from build123d import *

# Parameters (mm, degrees)
SKETCH3_R   = 14.887575
SKETCH3_R_2 = 10.4648
FILLET1_R   = 4.422775


with BuildPart() as part:
    # Sketch1 → Revolve1 (revolve)
    with BuildSketch(Plane.XY):
        Polygon((-26.19375, -17.859375), (-23.22195, -14.887575), (-23.22195, -10.4648), (-26.19375, -13.2842), (-51.59375, -13.4366), (-51.59375, -17.859375), align=None)
    revolve(axis=Axis((-51.59375, 0, 0), (1, 0, 0)))



with BuildPart() as body_2:
    # Sketch2 → Revolve2 (revolve)
    with BuildSketch(Plane.XY):
        Polygon((13.4366, 51.59375), (13.2842, 26.19375), (10.4648, 23.22195), (14.887575, 23.22195), (17.859375, 26.19375), (17.859375, 51.59375), align=None)
    revolve(axis=Axis((0, 0, 0), (0, 1, 0)))


with BuildPart() as part_1:
    add(part.part)

    add(body_2.part)  # Sweep1 merges body 2
    # Sweep1: sweep along a path in Sketch4
    with BuildLine(Plane.XY) as sweep1_path:
        ThreePointArc((-23.22195, 0), (-6.801551683, 6.801551683), (0, 23.22195))
    # Sketch3 → Sweep1 (sweep)
    with BuildSketch(Plane(origin=(-23.22195, 0, 0), x_dir=(0, 0, -1), z_dir=(1, 0, 0))):
        Circle(SKETCH3_R)
        Circle(SKETCH3_R_2, mode=Mode.SUBTRACT)
    sweep(path=sweep1_path.line)

    # Fillet1
    fillet1_edges = [part_1.edges().sort_by_distance(p)[0] for p in [
        (-23.22195, 10.527105238, 10.527105238),
        (-10.527105238, 23.22195, 10.527105238),
        (-17.859375, 26.19375, 0),
        (-26.19375, 17.859375, 0),
    ]]
    fillet(fillet1_edges, radius=FILLET1_R)


solid = part_1.part
Read the model definition and answer for the solid it produces. Units are mm, in the model's axes. A direction names the side the tool comes from. Give positions to 0.01 mm unless a question says otherwise; leave off trailing zeros. Write each loop counter-clockwise with the first axis right and the second up, starting at its lowest first coordinate (ties: lowest second). Pieces come first, ordered by that corner, then holes. Notation, with made-up numbers: (65, 1) - (116, 1) arc R22 ccw to (116, 40) - close; hole circle Ø11 at (14, -19.75). An arc over 180 degrees is marked (long way). Answer in a Markdown table with one row per item. Add a question column.
Item 1: Section A-A, the plane x = -34.5 is taken. Write down the section's boundary in (y, z), and give its area (3 significant figures).
Item 2: A tool of negligible diameter and unlimited length cuts with its end or side. For faces 5 (the face through (15.511, 24.596, -4.885)), 6 (the face through (16.498, 39.975, 6.84)), 7 (the face through (-39.645, -17.035, -5.364)), from which of +Z, -Z, +X, -X, +Y, -Y can it reach the whole face along a straight path? Write none if from no direction.
Item 3: Find the intervals of material crossed by L1, parallel to X at y = 15.5, z = -7; L2, parallel to X at y = 30, z = 10; L3, parallel to Y at x = -41.5, z = 3.5, in increasing order.
Item 4: Determine the mould class of faces 1 (the face through (-2.298, 23.366, 10.35)), 2 (the face through (-39.072, -12.744, -4.013)), 3 (the face through (-51.594, -7, -12)), 4 (the face through (-23.41, -10.15, -3.2)) for opening direction Y: pulls with the +Y half, pulls with the -Y half, needs draft (parallel to the pull), parting line crosses it, or undercut.
Item 5: Flat-ended cylindrical pins translate along their axes: P1, Ø1.5, axis at y = 30.5, z = 8, coming from the +X side; P2, Ø5, axis at x = 0, z = 10.5, coming from the +Y side; P3, Ø10, axis at x = -12, z = -14, coming from the +Y side; P4, Ø8, axis at y = 31, z = -2, coming from the -X side. Find the tip coordinate at first contact, or state that the pin passes through.
Recorded:
| question | item | result |
|---|---|---|
| 1 | outline | circle Ø35.72 at (0, 0); hole circle Ø26.67 at (0, 0) |
| 1 | area | 443 mm2 |
| 2 | face 5 | none |
| 2 | face 6 | +Y |
| 2 | face 7 | -X |
| 3 | L1 | x = -51.59 to -25.42, -16.74 to -9.85, 6.8 to 12.31 |
| 3 | L2 | x = -14.8 to -8.78, 8.78 to 14.8 |
| 3 | L3 | y = -17.51 to -12.91, 12.91 to 17.51 |
| 4 | face 1 | pulls with the +Y half |
| 4 | face 2 | undercut |
| 4 | face 3 | needs draft |
| 4 | face 4 | undercut |
| 5 | P1 | stops at x = 16.32 |
| 5 | P2 | stops at y = 25.89 |
| 5 | P3 | stops at y = 51.59 |
| 5 | P4 | stops at x = -17.86 |
